Autodesk Inventor part; units mm, degrees
ref_plane "YZ Plane" through (0, 0, 0) normal (1, 0, 0) x (0, 1, 0)
ref_plane "XZ Plane" through (0, 0, 0) normal (0, 1, 0) x (-1, 0, 0)
ref_plane "XY Plane" through (0, 0, 0) normal (0, 0, 1) x (1, 0, 0)
sketch "Skizze1" plane through (0, 0, 0) normal (0, 1, 0) x (-1, 0, 0)
  line L0 (17, 1) -> (22, 1)
  line L1 (22, 1) -> (22, 0)
  line L2 (22, 0) -> (0, 0)
  line L3 (0, 12.5) -> (0, 0)
  line L4 (99.15, 0) -> (-16.525, 0)
  line L5 (0, -2.5) -> (0, 15)
  line L6 (16, 12.5) -> (0, 12.5)
  arc A0 (16, 12.5) -> (17, 1) centre (82.625, 12.5) ccw
  line L7 (16, 12.5) -> (16, 0) construction
  dimension "d6" = 12.5
  dimension "d7" = 1
  dimension "d15" = 16
  dimension "d16" = 17
  dimension "d21" = 22
revolve "Umdrehung1" add sketch "Skizze1" angle 360 about axis through (0, 0, 12.5) along (0, 0, -1)
sketch "Skizze3" plane through (0, 0, 12.5) normal (0, 0, 1) x (1, 0, 0)
  circle A0 centre (0, 0) radius 22
  circle A1 centre (0, 0) radius 5.075
  dimension "d8" = 10.15
extrude "Extrusion2" cut sketch "Skizze3" against normal through all contours A1
sketch "Skizze4" plane through (0, 0, 12.5) normal (0, 0, 1) x (1, 0, 0)
  circle A0 centre (0, 0) radius 5.075
  circle A1 centre (0, 0) radius 16
  line L0 (-7.575, -7.575) -> (7.575, -7.575)
  line L1 (7.575, -7.575) -> (7.575, 7.575)
  line L2 (7.575, 7.575) -> (-7.575, 7.575)
  line L3 (-7.575, 7.575) -> (-7.575, -7.575)
  line L4 (-7.575, -7.575) -> (7.575, 7.575) construction
  line L5 (7.575, -7.575) -> (-7.575, 7.575) construction
  dimension "d11" = 15.15
  dimension "d12" = 15.15
extrude "Extrusion3" cut sketch "Skizze4" against normal blind 2.2 contours L3 L2 L1 L0
sketch "Skizze5" plane through (0, 0, 0) normal (0, 0, -1) x (-1, 0, 0)
  circle A0 centre (0, 0) radius 5.075
  circle A1 centre (0, 0) radius 22
  line L0 (-7.575, -7.575) -> (7.575, -7.575)
  line L1 (7.575, -7.575) -> (7.575, 7.575)
  line L2 (7.575, 7.575) -> (-7.575, 7.575)
  line L3 (-7.575, 7.575) -> (-7.575, -7.575)
  line L4 (-7.575, -7.575) -> (7.575, 7.575) construction
  line L5 (7.575, -7.575) -> (-7.575, 7.575) construction
  dimension "d17" = 15.15
  dimension "d18" = 15.15
extrude "Extrusion4" cut sketch "Skizze5" against normal blind 2.5 contours L3 L2 L1 L0
sketch "Skizze6" plane through (0, 0, 10.3) normal (0, 0, 1) x (1, 0, 0)
  line L0 (7.575, 7.575) -> (7.575, -7.575)
  line L1 (-7.575, 7.575) -> (7.575, 7.575)
  line L2 (-7.575, -7.575) -> (-7.575, 7.575)
  line L3 (7.575, -7.575) -> (-7.575, -7.575)
  circle A0 centre (0, 0) radius 5.075
extrude "Extrusion5" cut sketch "Skizze6" against normal through all
properties part number "Seil_Rolle_Antrieb_Mitte" material "PC/ABS-Kunststoff"
For this review, take the finished solid that the model builds, in its own axes (mm). A direction names the side the tool comes from. Round coordinates to 2 decimals unless told otherwise and drop trailing zeros. Write each loop counter-clockwise with the first axis right and the second up, starting at its lowest first coordinate (ties: lowest second). Pieces come first, ordered by that corner, then holes. Notation, with made-up numbers: (30.25, 31.5) -> (68.25, 31.5) arc R28 cw to (68.25, 52.5) -> close; hole circle Ø9 at (-32, -28). An arc over 180 degrees is marked (long way). One line per question, with ' | ' between items. Start each with the question number.
1) Add section A-A (x = 0). Write out the cut boundary in (y, z) (3 decimals), and give its area (3 significant figures).
2) Mouldability with a two-part tool opening along X and no side actions: class faces 1 (the flat face through (0, -7.575, 6)), 2 (the flat face through (-10, 0, 12.5)), 3 (the flat face through (7.575, 0, 6)), 4 (the cylindrical face through (4.769, -21.477, 0.493)) as +X half, -X half, draft (parallel to the pull), parting line (faces both ways), or undercut.
3) Wall thickness on line 1 along X through (y, z) = (6.5, 10) (3 decimals); line 2 along X through (y, z) = (-1, 5.5) (3 decimals); line 3 along Y through (x, z) = (1, 10) (3 decimals): over which ranges is each line inside the solid? List them lowest first.
4) Machinability: for faces 5 (the flat face through (0, 7.575, 6)), 6 (the flat face through (0, -9, 0)), 7 (the flat face through (-11.3, -12.93, 1)), which of the approach directions +Z, -Z, +X, -X, +Y, -Y give a long, thin tool a straight path to every point of the face, cutting with its end or side? Answer none if there is none.
5) Add section D-D (y = 18.5). Write out the cut boundary in (x, z), and give its area (3 significant figures).
6) For pin 1 Ø6 at (x, z) = (1, 6) entering from +Y; pin 2 Ø2 at (x, z) = (7, 6.5) entering from -Y; pin 3 Ø6 at (y, z) = (-10, 6) entering from +X, all flat-tipped, find the tip position at first contact; note any pin that passes through.
7) Add section C-C (z = 4.75). Write out the cut boundary in (x, y) (3 decimals), and give its area (3 significant figures).
Reported:
1) outline: (-22, 0) -> (-7.575, 0) -> (-7.575, 12.5) -> (-16, 12.5) arc R66.625 cw to (-17, 1) -> (-22, 1) -> close; (7.575, 0) -> (22, 0) -> (22, 1) -> (17, 1) arc R66.625 cw to (16, 12.5) -> (7.575, 12.5) -> close | area: 230 mm²
2) face 1: undercut | face 2: draft | face 3: undercut | face 4: parting line
3) line 1: x = -14.672 to -7.575, 7.575 to 14.672 | line 2: x = -16.338 to -7.575, 7.575 to 16.338 | line 3: y = -16.016 to -7.575, 7.575 to 16.016
4) face 5: +Z, -Z | face 6: -Z, +X, -X, +Y, -Y | face 7: +Z
5) outline: (-11.91, 0) -> (11.91, 0) -> (11.91, 1) -> (-11.91, 1) -> close | area: 23.8 mm²
6) pin 1: stops at y = 16.67 | pin 2: stops at y = -15.14 | pin 3: stops at x = 14.78
7) outline: circle Ø32.905 at (0, 0); hole (-7.575, -7.575) -> (7.575, -7.575) -> (7.575, 7.575) -> (-7.575, 7.575) -> close | area: 621 mm²
